Source: CAD feature listing. Evaluate the final solid. Frame: model axes, mm. Round coordinates to 2 decimals unless told otherwise and drop trailing zeros. Loops run counter-clockwise (first coordinate to the right, second up) from the corner with the lowest first, then second, coordinate; pieces in that order, holes last. Notation, with made-up numbers: (-1, 47) -> (43, 47) arc R11 ccw to (43, 56) -> close; hole circle Ø5 at (-3.5, 88.25). An arc over 180 degrees is marked (long way). Put each result on its own line as item: value. Start each with the question number.
1. Cut plane C-C (y = 26). Return the cut outline in (x, z) (3 decimals).
2. Cut plane A-A (z = 1.95). State how many separate pieces and enclosed holes the cut face has, then the cut area to 3 significant figures.
3. Contact query for flat-ended pins moving along their axis: pin 1 (2.5 mm diameter, centred on x = 41.46, y = 16.49, fed in from +Z); pin 2 (1.5 mm diameter, centred on x = -34.5, z = 0.5, fed in from +Y); pin 3 (1.5 mm diameter, centred on y = 31.5, z = 3, fed in from -X). Output: stop coordinate, or through.
4. Cut plane B-B (x = -29). Return the cut outline in (y, z) (3 decimals).
5. Draft query along Y for faces 1 (the flat face through (0, 46.228, 2)), 2 (the flat face through (-46.228, 0, 2)), 3 (the cylindrical face through (-16.97, 39.33, 1.61)). Return one class per face: pulls with the +Y half, pulls with the -Y half, needs draft (parallel to the pull), parting line crosses it, or undercut.
6. Material intervals for L1, parallel to X at y = -40, z = 0.95; L2, parallel to X at y = 18, z = 2.85; L3, parallel to Y at x = -17.5, z = 0.8, sorted ascending.
```python
from build123d import *

# Parameters (mm, degrees)
BOSS_EXTRUDE1_DEPTH = 3.175
CUT_EXTRUDE2_REACH  = 69.068
SKETCH3_R           = 2.1828125
SKETCH4_W           = 109.59125296
SKETCH4_H           = 128.097404578
CUT_EXTRUDE3_DEPTH  = 68.067905193


with BuildPart() as part:
    # Sketch1 → Boss-Extrude1 (new body)
    with BuildSketch(Plane.XY):
        with BuildLine():
            Line((46.57725, -47.371), (-46.57725, -47.371))
            ThreePointArc((-46.57725, -47.371), (-47.138516008, -47.138516008), (-47.371, -46.57725))
            Line((-47.371, -46.57725), (-47.371, 46.57725))
            ThreePointArc((-47.371, 46.57725), (-47.138516008, 47.138516008), (-46.57725, 47.371))
            Line((-46.57725, 47.371), (46.57725, 47.371))
            ThreePointArc((46.57725, 47.371), (47.138516008, 47.138516008), (47.371, 46.57725))
            Line((47.371, 46.57725), (47.371, -46.57725))
            ThreePointArc((47.371, -46.57725), (47.138516008, -47.138516008), (46.57725, -47.371))
        make_face()
    extrude(amount=BOSS_EXTRUDE1_DEPTH)

    # Sketch3 → Cut-Extrude2 (cut, up to next)
    with BuildSketch(Plane.XY.offset(3.175), mode=Mode.PRIVATE) as cut_extrude2_sk1:
        with Locations((16.490011722, -41.462970183)):
            Circle(SKETCH3_R)
    cut_extrude2_tool1 = extrude(cut_extrude2_sk1.sketch, amount=-CUT_EXTRUDE2_REACH, mode=Mode.PRIVATE) & part.part
    # Sketch3 → Cut-Extrude2 (cut, up to next)
    with BuildSketch(Plane.XY.offset(3.175), mode=Mode.PRIVATE) as cut_extrude2_sk2:
        with Locations((34.1474239, -34.1474239)):
            Circle(SKETCH3_R)
    cut_extrude2_tool2 = extrude(cut_extrude2_sk2.sketch, amount=-CUT_EXTRUDE2_REACH, mode=Mode.PRIVATE) & part.part
    # Sketch3 → Cut-Extrude2 (cut, up to next)
    with BuildSketch(Plane.XY.offset(3.175), mode=Mode.PRIVATE) as cut_extrude2_sk3:
        with Locations((41.460741539, -16.494469011)):
            Circle(SKETCH3_R)
    cut_extrude2_tool3 = extrude(cut_extrude2_sk3.sketch, amount=-CUT_EXTRUDE2_REACH, mode=Mode.PRIVATE) & part.part
    # Sketch3 → Cut-Extrude2 (cut, up to next)
    with BuildSketch(Plane.XY.offset(3.175), mode=Mode.PRIVATE) as cut_extrude2_sk4:
        with Locations((41.460741539, 16.490011722)):
            Circle(SKETCH3_R)
    cut_extrude2_tool4 = extrude(cut_extrude2_sk4.sketch, amount=-CUT_EXTRUDE2_REACH, mode=Mode.PRIVATE) & part.part
    # Sketch3 → Cut-Extrude2 (cut, up to next)
    with BuildSketch(Plane.XY.offset(3.175), mode=Mode.PRIVATE) as cut_extrude2_sk5:
        with Locations((34.335639739, 33.869270843)):
            Circle(SKETCH3_R)
    cut_extrude2_tool5 = extrude(cut_extrude2_sk5.sketch, amount=-CUT_EXTRUDE2_REACH, mode=Mode.PRIVATE) & part.part
    # Sketch3 → Cut-Extrude2 (cut, up to next)
    with BuildSketch(Plane.XY.offset(3.175), mode=Mode.PRIVATE) as cut_extrude2_sk6:
        with Locations((16.492240366, 41.460741539)):
            Circle(SKETCH3_R)
    cut_extrude2_tool6 = extrude(cut_extrude2_sk6.sketch, amount=-CUT_EXTRUDE2_REACH, mode=Mode.PRIVATE) & part.part
    # Sketch3 → Cut-Extrude2 (cut, up to next)
    with BuildSketch(Plane.XY.offset(3.175), mode=Mode.PRIVATE) as cut_extrude2_sk7:
        with Locations((-16.492240366, 41.460741539)):
            Circle(SKETCH3_R)
    cut_extrude2_tool7 = extrude(cut_extrude2_sk7.sketch, amount=-CUT_EXTRUDE2_REACH, mode=Mode.PRIVATE) & part.part
    # Sketch3 → Cut-Extrude2 (cut, up to next)
    with BuildSketch(Plane.XY.offset(3.175), mode=Mode.PRIVATE) as cut_extrude2_sk8:
        with Locations((-33.681055005, 34.057486682)):
            Circle(SKETCH3_R)
    cut_extrude2_tool8 = extrude(cut_extrude2_sk8.sketch, amount=-CUT_EXTRUDE2_REACH, mode=Mode.PRIVATE) & part.part
    # Sketch3 → Cut-Extrude2 (cut, up to next)
    with BuildSketch(Plane.XY.offset(3.175), mode=Mode.PRIVATE) as cut_extrude2_sk9:
        with Locations((-41.462970183, 16.492240366)):
            Circle(SKETCH3_R)
    cut_extrude2_tool9 = extrude(cut_extrude2_sk9.sketch, amount=-CUT_EXTRUDE2_REACH, mode=Mode.PRIVATE) & part.part
    # Sketch3 → Cut-Extrude2 (cut, up to next)
    with BuildSketch(Plane.XY.offset(3.175), mode=Mode.PRIVATE) as cut_extrude2_sk10:
        with Locations((-41.462970183, -16.492240366)):
            Circle(SKETCH3_R)
    cut_extrude2_tool10 = extrude(cut_extrude2_sk10.sketch, amount=-CUT_EXTRUDE2_REACH, mode=Mode.PRIVATE) & part.part
    # Sketch3 → Cut-Extrude2 (cut, up to next)
    with BuildSketch(Plane.XY.offset(3.175), mode=Mode.PRIVATE) as cut_extrude2_sk11:
        with Locations((-16.494469011, -41.462970183)):
            Circle(SKETCH3_R)
    cut_extrude2_tool11 = extrude(cut_extrude2_sk11.sketch, amount=-CUT_EXTRUDE2_REACH, mode=Mode.PRIVATE) & part.part
    # Sketch3 → Cut-Extrude2 (cut, up to next)
    with BuildSketch(Plane.XY.offset(3.175), mode=Mode.PRIVATE) as cut_extrude2_sk12:
        with Locations((-33.869270843, -33.959208062)):
            Circle(SKETCH3_R)
    cut_extrude2_tool12 = extrude(cut_extrude2_sk12.sketch, amount=-CUT_EXTRUDE2_REACH, mode=Mode.PRIVATE) & part.part
    add(cut_extrude2_tool1.solids().sort_by_distance((16.490012, -41.46297, 3.175))[0], mode=Mode.SUBTRACT)
    add(cut_extrude2_tool2.solids().sort_by_distance((34.147424, -34.147424, 3.175))[0], mode=Mode.SUBTRACT)
    add(cut_extrude2_tool3.solids().sort_by_distance((41.460742, -16.494469, 3.175))[0], mode=Mode.SUBTRACT)
    add(cut_extrude2_tool4.solids().sort_by_distance((41.460742, 16.490012, 3.175))[0], mode=Mode.SUBTRACT)
    add(cut_extrude2_tool5.solids().sort_by_distance((34.33564, 33.869271, 3.175))[0], mode=Mode.SUBTRACT)
    add(cut_extrude2_tool6.solids().sort_by_distance((16.49224, 41.460742, 3.175))[0], mode=Mode.SUBTRACT)
    add(cut_extrude2_tool7.solids().sort_by_distance((-16.49224, 41.460742, 3.175))[0], mode=Mode.SUBTRACT)
    add(cut_extrude2_tool8.solids().sort_by_distance((-33.681055, 34.057487, 3.175))[0], mode=Mode.SUBTRACT)
    add(cut_extrude2_tool9.solids().sort_by_distance((-41.46297, 16.49224, 3.175))[0], mode=Mode.SUBTRACT)
    add(cut_extrude2_tool10.solids().sort_by_distance((-41.46297, -16.49224, 3.175))[0], mode=Mode.SUBTRACT)
    add(cut_extrude2_tool11.solids().sort_by_distance((-16.494469, -41.46297, 3.175))[0], mode=Mode.SUBTRACT)
    add(cut_extrude2_tool12.solids().sort_by_distance((-33.869271, -33.959208, 3.175))[0], mode=Mode.SUBTRACT)

    # Sketch4 → Cut-Extrude3 (cut, through all)
    with BuildSketch(Plane.XY.offset(3.175)):
        Rectangle(SKETCH4_W, SKETCH4_H)
        with BuildLine():
            Line((16.4846, -46.228), (-16.4846, -46.228))
            ThreePointArc((-16.4846, -46.228), (-37.516359836, -37.516359836), (-46.228, -16.4846))
            Line((-46.228, -16.4846), (-46.228, 16.4846))
            ThreePointArc((-46.228, 16.4846), (-37.516359836, 37.516359836), (-16.4846, 46.228))
            Line((-16.4846, 46.228), (16.4846, 46.228))
            ThreePointArc((16.4846, 46.228), (37.516359836, 37.516359836), (46.228, 16.4846))
            Line((46.228, 16.4846), (46.228, -16.4846))
            ThreePointArc((46.228, -16.4846), (37.516359836, -37.516359836), (16.4846, -46.228))
        make_face(mode=Mode.SUBTRACT)
    extrude(amount=-CUT_EXTRUDE3_DEPTH, mode=Mode.SUBTRACT)


solid = part.part
```
Solution:
1. outline: (-44.665, 0) -> (44.665, 0) -> (44.665, 3.175) -> (-44.665, 3.175) -> close
2. separate pieces: 1
2. enclosed holes: 12
2. area: 7,610 mm^2
3. pin 1: passes through
3. pin 2: stops at y = 40.7
3. pin 3: stops at x = -42.58
4. outline: (-43.467, 0) -> (43.467, 0) -> (43.467, 3.175) -> (-43.467, 3.175) -> close
5. face 1: pulls with the +Y half
5. face 2: needs draft
5. face 3: undercut
6. L1: x = -34.7 to -18.11, -14.87 to 14.87, 18.11 to 34.7
6. L2: x = -46.19 to -43.04, -39.88 to 39.88, 43.04 to 46.19
6. L3: y = -46.21 to -43.4, -39.53 to 39.52, 43.4 to 46.21
